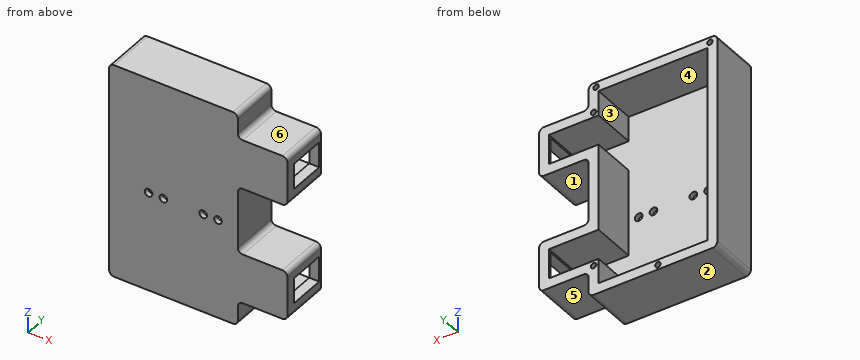
```python
from build123d import *

# Parameters (mm, degrees)
BOSS_EXTRUDE1_DEPTH = 20
SKETCH2_W           = 44
SKETCH2_H           = 79
CUT_EXTRUDE1_DEPTH  = 18
SKETCH3_W           = 20
SKETCH3_H           = 12
CUT_EXTRUDE2_DEPTH  = 18
SKETCH4_R           = 1.1
CUT_EXTRUDE3_DEPTH  = 10
SKETCH5_R           = 1.1
CUT_EXTRUDE4_DEPTH  = 10
SKETCH6_W           = 10.3
SKETCH6_H           = 15
CUT_EXTRUDE5_DEPTH  = 6
SKETCH7_R           = 1.55
CUT_EXTRUDE6_DEPTH  = 6
FILLET1_R           = 2


with BuildPart() as part:
    # Sketch1 → Boss-Extrude1 (new body)
    with BuildSketch(Plane(origin=(0, 0, 0), x_dir=(1, 0, 0), z_dir=(0, 1, 0))):
        Polygon((53.327223789, 77.96478334), (53.327223789, 87.96478334), (1.327223789, 87.96478334), (1.327223789, 0.96478334), (53.327223789, 0.96478334), (53.327223789, 10.96478334), (73.327223789, 10.96478334), (73.327223789, 30.96478334), (53.327223789, 30.96478334), (53.327223789, 57.96478334), (73.327223789, 57.96478334), (73.327223789, 77.96478334), align=None)
    extrude(amount=BOSS_EXTRUDE1_DEPTH)

    # Sketch2 → Cut-Extrude1 (cut)
    with BuildSketch(Plane(origin=(0, 20, 0), x_dir=(1, 0, 0), z_dir=(0, 1, 0))):
        with Locations((27.327223789, 44.46478334)):
            Rectangle(SKETCH2_W, SKETCH2_H)
    extrude(amount=-CUT_EXTRUDE1_DEPTH, mode=Mode.SUBTRACT)

    # Sketch3 → Cut-Extrude2 (cut)
    with BuildSketch(Plane(origin=(0, 20, 0), x_dir=(1, 0, 0), z_dir=(0, 1, 0))):
        with Locations((59.327223789, 67.96478334)):
            Rectangle(SKETCH3_W, SKETCH3_H)
        with Locations((59.327223789, 20.96478334)):
            Rectangle(SKETCH3_W, SKETCH3_H)
    extrude(amount=-CUT_EXTRUDE2_DEPTH, mode=Mode.SUBTRACT)

    # Sketch4 → Cut-Extrude3 (cut)
    with BuildSketch(Plane(origin=(0, 20, 0), x_dir=(1, 0, 0), z_dir=(0, 1, 0))):
        with Locations((4.327223789, 2.96478334)):
            Circle(SKETCH4_R)
        with Locations((50.327223789, 2.96478334)):
            Circle(SKETCH4_R)
        with Locations((25.327223789, 85.96478334)):
            Circle(SKETCH4_R)
    extrude(amount=-CUT_EXTRUDE3_DEPTH, mode=Mode.SUBTRACT)

    # Sketch5 → Cut-Extrude4 (cut)
    with BuildSketch(Plane(origin=(0, 20, 0), x_dir=(1, 0, 0), z_dir=(0, 1, 0))):
        with Locations((51.327223789, 12.96478334)):
            Circle(SKETCH5_R)
        with Locations((51.327223789, 75.96478334)):
            Circle(SKETCH5_R)
    extrude(amount=-CUT_EXTRUDE4_DEPTH, mode=Mode.SUBTRACT)

    # Sketch6 → Cut-Extrude5 (cut)
    with BuildSketch(Plane(origin=(73.327223789, 0, 0), x_dir=(0, 0, -1), z_dir=(1, 0, 0))):
        with Locations((67.96478334, 11.5)):
            Rectangle(SKETCH6_W, SKETCH6_H)
        with Locations((20.96478334, 11.5)):
            Rectangle(SKETCH6_W, SKETCH6_H)
    extrude(amount=-CUT_EXTRUDE5_DEPTH, mode=Mode.SUBTRACT)

    # Sketch7 → Cut-Extrude6 (cut)
    with BuildSketch(Plane(origin=(0, 2, 0), x_dir=(1, 0, 0), z_dir=(0, 1, 0))):
        with Locations((45.297223789, 47.81478334)):
            Circle(SKETCH7_R)
        with Locations((23.237223789, 47.81478334)):
            Circle(SKETCH7_R)
        with Locations((39.327223789, 47.81478334)):
            Circle(SKETCH7_R)
        with Locations((17.267223789, 47.81478334)):
            Circle(SKETCH7_R)
    extrude(amount=-CUT_EXTRUDE6_DEPTH, mode=Mode.SUBTRACT)

    # Fillet1
    fillet1_edges = [part.edges().sort_by_distance(p)[0] for p in [
        (1.327223789, 10, -87.96478334),
        (53.327223789, 10, -87.96478334),
        (53.327223789, 10, -77.96478334),
        (73.327223789, 10, -77.96478334),
        (73.327223789, 10, -57.96478334),
        (53.327223789, 10, -57.96478334),
        (53.327223789, 10, -30.96478334),
        (73.327223789, 10, -30.96478334),
        (73.327223789, 10, -10.96478334),
        (53.327223789, 10, -10.96478334),
        (53.327223789, 10, -0.96478334),
        (1.327223789, 10, -0.96478334),
    ]]
    fillet(fillet1_edges, radius=FILLET1_R)


solid = part.part
```
Verification items for the finished model (mm, model axes). Face numbers are marked on the shaded views. A direction names the side the tool comes from. Coordinates: 2 decimals unless noted, no trailing zeros. Order: outer loops, then holes, each group sorted by start corner. A loop starts at its lowest first (then second) coordinate and runs counter-clockwise, first axis right, second up. Notation, with made-up numbers: (88.5, -1) -> (121.5, -1) arc R29 cw to (121.5, 20) -> close; hole circle Ø3 at (45.5, 26.5). An arc over 180 degrees is marked (long way). Answer as CSV lines item,"result". Start each with the question number.
1) Set-up check for the marked faces 1, 2 and 3: record each of +Z, -Z, +X, -X, +Y, -Y from which the full face is reachable in a straight line by a thin tool's end or side.
2) Cross-section at C-C, the plane x = 13. Record the boundary of the cut face in (y, z).
3) Gauge pin test, flat ends, axial feed: pin 1 Ø3 at (x, z) = (41.5, -52) entering from +Y; pin 2 Ø1.1 at (x, z) = (25.5, -85.5) entering from +Y; pin 3 Ø3 at (x, z) = (71, -19) entering from -Y; pin 4 Ø2.5 at (x, z) = (45.3, -47.81) entering from +Y. Record the tip position at first contact, or that the pin passes through.
4) Cross-section at B-B, the plane y = 11. Give the number of separate pieces and of enclosed holes in the cut face, then the cut area to 3 significant figures.
5) Cross-section at A-A, the plane x = 63. Record the boundary of the cut face in (y, z).
6) Release check for a two-part mould opening along Z. For the marked faces 4, 5 and 6 record: released by +Z, released by -Z, zero draft, split by the parting line, or undercut.
7) Cross-section at D-D, the plane z = -36. Record the boundary of the cut face in (x, y).
8) Material ranges on L1, parallel to Z at x = 67, y = 8.5; L2, parallel to Z at x = 9, y = 17.25; L3, parallel to X at y = 5, z = -26.5, recorded low to high. Write a range as [from, to].
Conclusion:
1,face 1,"+X, +Y, -Y"
1,face 2,"-Z, +X, -X, +Y, -Y"
1,face 3,"+Y"
2,outline,"(0, -87.96) -> (20, -87.96) -> (20, -83.96) -> (2, -83.96) -> (2, -4.96) -> (20, -4.96) -> (20, -0.96) -> (0, -0.96) -> close"
3,pin 1,"stops at y = 2"
3,pin 2,"stops at y = 10"
3,pin 3,"stops at y = 0"
3,pin 4,"passes through"
4,separate pieces,"2"
4,enclosed holes,"5"
4,area,"1,260 mm²"
5,outline,"(0, -77.96) -> (20, -77.96) -> (20, -73.96) -> (2, -73.96) -> (2, -61.96) -> (20, -61.96) -> (20, -57.96) -> (0, -57.96) -> close; (0, -30.96) -> (20, -30.96) -> (20, -26.96) -> (2, -26.96) -> (2, -14.96) -> (20, -14.96) -> (20, -10.96) -> (0, -10.96) -> close"
6,face 4,"undercut"
6,face 5,"released by -Z"
6,face 6,"released by +Z"
7,outline,"(1.33, 0) -> (53.33, 0) -> (53.33, 20) -> (49.33, 20) -> (49.33, 2) -> (5.33, 2) -> (5.33, 20) -> (1.33, 20) -> close"
8,L1,"z = [-77.96, -73.96], [-61.96, -57.96], [-30.96, -26.96], [-14.96, -10.96]"
8,L2,"z = [-87.96, -83.96], [-4.96, -0.96]"
8,L3,"x = [1.33, 5.33], [69.33, 73.33]"
